Source: CAD feature listing. Evaluate the final solid. Frame: model axes, mm. A direction names the side the tool comes from. Round coordinates to 2 decimals unless told otherwise and drop trailing zeros. Order: outer loops, then holes, each group sorted by start corner. A loop starts at its lowest first (then second) coordinate and runs counter-clockwise, first axis right, second up. Notation, with made-up numbers: (-3.5, 49) -> (37.5, 49) arc R22 ccw to (37.5, 59) -> close; hole circle Ø10 at (-10.5, 77.25). An arc over 180 degrees is marked (long way). Answer as CSV lines item,"result". Start each with the question number.
(1) Section query B-B (x = 53.5). Output: boundary loops of the cut face in (y, z), plus the area to 3 significant figures.
(2) Section query D-D (z = 50). Output: boundary loops of the cut face in (x, y).
(3) Section query C-C (x = 34). Output: boundary loops of the cut face in (y, z), plus the area to 3 significant figures.
(4) Pull-direction query (Z, two-part tool) for faces 1 (the flat face through (59, -52, 0)), 2 (the flat face through (49, 0, 44)), 3 (the cylindrical face through (99.5, -20.2, 81)); classes: +Z half, -Z half, draft (parallel to the pull), parting line (faces both ways), or undercut.
(5) Section query A-A (z = 77). Output: boundary loops of the cut face in (x, y), plus the area to 3 significant figures.
(6) Set-up query: faces 4 (the flat face through (97, -25, 44)), 5 (the cylindrical face through (6.09, -52.54, 7.9)). Return all of +Z, -Z, +X, -X, +Y, -Y with unobstructed straight access to the full face (end or side cutting, diameter ignored); none if empty.
(7) Line query: line 1 along X through (y, z) = (-51, 50); line 2 along Y through (x, z) = (24.5, 80.5); line 3 along X through (y, z) = (-13, 66). Output: solid intervals per line, ascending. Write a range as from..to.
(8) Contact query for flat-ended pins moving along their axis: P1, Ø2.5, axis at x = 6, z = 10, coming from the +Y side; P2, Ø4, axis at y = -5.25, z = 83.42, coming from the +X side; P3, Ø4, axis at y = -10.19, z = 67.73, coming from the -X side. Output: stop coordinate, or through.
```python
from build123d import *

# Parameters (mm, degrees)
EXTRUDE_1_DEPTH          = 90
CUT_EXTRUDE1_DEPTH       = 147.727638841
CUT_EXTRUDE1_DEPTH_BACK  = 147.727638841
SKETCH1_R                = 2.1
SKETCH_2_R               = 7
CUT_EXTRUDE_1_DEPTH      = 10
SKETCH_6_R               = 1.6
CUT_EXTRUDE_3_DEPTH      = 10
PATTERN_CIRCULAR_1_COUNT = 3


with BuildPart() as part:
    # 草图1 → 凸台-拉伸1 (new body)
    with BuildSketch(Plane.XY):
        Polygon((0, 0), (0, 5), (102, 5), (102, -55), (0, -55), (0, -50), (97, -50), (97, 0), align=None)
    extrude(amount=EXTRUDE_1_DEPTH)

    # Sketch1 → Cut-Extrude1 (cut, two sides: drawn at the far end of the back side and taken through both)
    with BuildSketch(Plane(origin=(0, 0, 0), x_dir=(1, 0, 0), z_dir=(0, 1, 0)).offset(-CUT_EXTRUDE1_DEPTH_BACK)):
        with Locations(Location((6, -10, 0), (0, 0, 270))):
            Circle(SKETCH1_R)
        with Locations(Location((34, -10, 0), (0, 0, 270))):
            Circle(SKETCH1_R)
        with Locations(Location((34, -50, 0), (0, 0, 270))):
            Circle(SKETCH1_R)
        with Locations(Location((6, -50, 0), (0, 0, 270))):
            Circle(SKETCH1_R)
    extrude(amount=CUT_EXTRUDE1_DEPTH + CUT_EXTRUDE1_DEPTH_BACK, mode=Mode.SUBTRACT)

    # 草图2 → 切除-拉伸1 (cut)
    with BuildSketch(Plane.ZY.offset(-97)):
        with Locations((77, -12.25)):
            Circle(SKETCH_2_R)
    extrude(amount=-CUT_EXTRUDE_1_DEPTH, mode=Mode.SUBTRACT)

    # 草图6 → 切除-拉伸3 (cut)
    with BuildSketch(Plane(origin=(102, 0, 0), x_dir=(0, 0, -1), z_dir=(1, 0, 0))):
        with Locations((-83.421648209, -5.249111894)):
            Circle(SKETCH_6_R)
    cut_extrude_3 = extrude(amount=-CUT_EXTRUDE_3_DEPTH, mode=Mode.SUBTRACT)

    # 阵列(圆周)1: 切除-拉伸3 ×3 about axis
    pattern_circular_1_axis = Axis((0, -12.25, 77), (1, 0, 0))
    for i in range(1, PATTERN_CIRCULAR_1_COUNT):
        add(cut_extrude_3.rotate(pattern_circular_1_axis, i * 360 / PATTERN_CIRCULAR_1_COUNT), mode=Mode.SUBTRACT)


solid = part.part
```
Answer block:
1,outline,"(-55, 0) -> (-50, 0) -> (-50, 90) -> (-55, 90) -> close; (0, 0) -> (5, 0) -> (5, 90) -> (0, 90) -> close"
1,area,"900 mm2"
2,outline,"(0, -55) -> (3.9, -55) -> (3.9, -50) -> (0, -50) -> close; (0, 0) -> (3.9, 0) -> (3.9, 5) -> (0, 5) -> close; (8.1, -55) -> (31.9, -55) -> (31.9, -50) -> (8.1, -50) -> close; (8.1, 0) -> (31.9, 0) -> (31.9, 5) -> (8.1, 5) -> close; (36.1, -55) -> (102, -55) -> (102, 5) -> (36.1, 5) -> (36.1, 0) -> (97, 0) -> (97, -50) -> (36.1, -50) -> close"
3,outline,"(-55, 0) -> (-50, 0) -> (-50, 7.9) -> (-55, 7.9) -> close; (-55, 12.1) -> (-50, 12.1) -> (-50, 47.9) -> (-55, 47.9) -> close; (-55, 52.1) -> (-50, 52.1) -> (-50, 90) -> (-55, 90) -> close; (0, 0) -> (5, 0) -> (5, 7.9) -> (0, 7.9) -> close; (0, 12.1) -> (5, 12.1) -> (5, 47.9) -> (0, 47.9) -> close; (0, 52.1) -> (5, 52.1) -> (5, 90) -> (0, 90) -> close"
3,area,"816 mm2"
4,face 1,"-Z half"
4,face 2,"draft"
4,face 3,"undercut"
5,outline,"(0, -55) -> (102, -55) -> (102, -19.25) -> (97, -19.25) -> (97, -50) -> (0, -50) -> close; (0, 0) -> (97, 0) -> (97, -5.25) -> (102, -5.25) -> (102, 5) -> (0, 5) -> close"
5,area,"1,200 mm2"
6,face 4,"+Z, -Z, -X"
6,face 5,"+Y, -Y"
7,line 1,"0..3.9, 8.1..31.9, 36.1..102"
7,line 2,"-55..-50, 0..5"
7,line 3,"97..102"
8,P1,"through"
8,P2,"x = 102"
8,P3,"x = 97"
